Autodesk Fusion 360 part; units mm, degrees
sketch "Sketch1" plane through (0, 0, 0) normal (0, 0, 1) x (1, 0, 0)
  line L0 (0, 0) -> (50.8, 0)
  line L1 (50.8, 0) -> (50.8, 50.8)
  line L2 (50.8, 50.8) -> (0, 50.8)
  line L3 (0, 50.8) -> (0, 0)
  dimension "d1" = 50.8
  dimension "d2" = 50.8
extrude "Extrude1" add sketch "Sketch1" along normal blind 31.75
sketch "Sketch2" plane through (50.8, 0, 0) normal (1, 0, 0) x (0, 1, 0)
  line L0 (0, 0) -> (50.8, 0)
  line L1 (50.8, 0) -> (50.8, 31.75)
  line L2 (50.8, 31.75) -> (0, 31.75)
  line L3 (0, 31.75) -> (0, 0)
  line L4 (50.8, 23.368) -> (10.16, 23.368)
  line L5 (10.16, 23.368) -> (10.16, 3.81)
  line L6 (10.16, 3.81) -> (50.8, 3.81)
  line L7 (50.8, 3.81) -> (50.8, 23.368)
  dimension "d5" = 40.64
  dimension "d6" = 19.558
  dimension "d14" = 3.81
extrude "Extrude2" cut sketch "Sketch2" against normal blind 40.64 contours L1 L4 L5 L6 L7
sketch "Sketch3" plane through (0, 0, 31.75) normal (0, 0, 1) x (-1, 0, 0)
  line L0 (0, -50.8) -> (0, 0)
  line L1 (0, 0) -> (-50.8, 0)
  line L2 (-50.8, 0) -> (-50.8, -50.8)
  line L3 (-50.8, -50.8) -> (0, -50.8)
  line L4 (0, 0) -> (-25.4, 0)
  line L5 (-25.4, 0) -> (-25.4, -25.4)
  line L6 (-25.4, -25.4) -> (0, -25.4)
  line L7 (0, -25.4) -> (0, 0)
  dimension "d10" = 25.4
  dimension "d11" = 25.4
extrude "Extrude3" add sketch "Sketch3" along normal blind 152.4 contours L0 L1 L4 L5 L6 L7
fillet "Fillet1" radius 2.54 2 edges at (25.4, 12.7, 31.75) (12.7, 25.4, 31.75)
sketch "Sketch4" plane through (0, 0, 0) normal (0, 0, -1) x (1, 0, 0)
  line L0 (0, 0) -> (0, -50.8)
  line L1 (0, -50.8) -> (50.8, -50.8)
  line L2 (50.8, -50.8) -> (50.8, 0)
  line L3 (50.8, 0) -> (0, 0)
  line L4 (2.54, -2.54) -> (22.86, -2.54)
  line L5 (22.86, -2.54) -> (22.86, -22.86)
  line L6 (22.86, -22.86) -> (2.54, -22.86)
  line L7 (2.54, -22.86) -> (2.54, -2.54)
  dimension "d17" = 2.54
  dimension "d18" = 2.54
  dimension "d19" = 20.32
  dimension "d20" = 20.32
sketch "Sketch5" plane through (0, 0, 0) normal (0, 0, -1) x (1, 0, 0)
  line L0 (5.08, -5.08) -> (20.32, -5.08)
  line L1 (20.32, -5.08) -> (20.32, -20.32)
  line L2 (20.32, -20.32) -> (5.08, -20.32)
  line L3 (5.08, -20.32) -> (5.08, -5.08)
  line L4 (2.54, -2.54) -> (22.86, -2.54)
  line L5 (2.54, -22.86) -> (2.54, -2.54)
  dimension "d21" = 2.54
  dimension "d22" = 2.54
  dimension "d23" = 15.24
  dimension "d24" = 15.24
extrude "Extrude4" add sketch "Sketch5" along normal blind 5.08
loft "Loft1" add profiles "Sketch4" section 1 contours L4 L5 L6 L7 section 2 face at (10.16, 15.24, -5.08)
sketch "Sketch6" plane through (0, 0, 184.15) normal (0, 0, 1) x (-1, 0, 0)
  line L0 (0, -25.4) -> (0, 0)
  line L1 (0, 0) -> (-25.4, 0)
  line L2 (-25.4, 0) -> (-25.4, -25.4)
  line L3 (-25.4, -25.4) -> (0, -25.4)
  line L4 (-2.54, -22.86) -> (-22.86, -22.86)
  line L5 (-22.86, -22.86) -> (-22.86, -2.54)
  line L6 (-22.86, -2.54) -> (-2.54, -2.54)
  line L7 (-2.54, -2.54) -> (-2.54, -22.86)
  line L8 (-5.08, -20.32) -> (-20.32, -20.32)
  line L9 (-20.32, -20.32) -> (-20.32, -5.08)
  line L10 (-20.32, -5.08) -> (-5.08, -5.08)
  line L11 (-5.08, -5.08) -> (-5.08, -20.32)
  dimension "d27" = 2.54
  dimension "d28" = 2.54
  dimension "d29" = 2.54
  dimension "d30" = 20.32
  dimension "d31" = 2.54
  dimension "d32" = 15.24
  dimension "d33" = 15.24
  dimension "d34" = 2.54
extrude "Extrude5" cut sketch "Sketch6" against normal blind 5.08 contours L8 L9 L10 L11
loft "Loft2" cut profiles "Sketch6" section 1 contours L4 L5 L6 L7 section 2 face at (15.24, 15.24, 179.07)
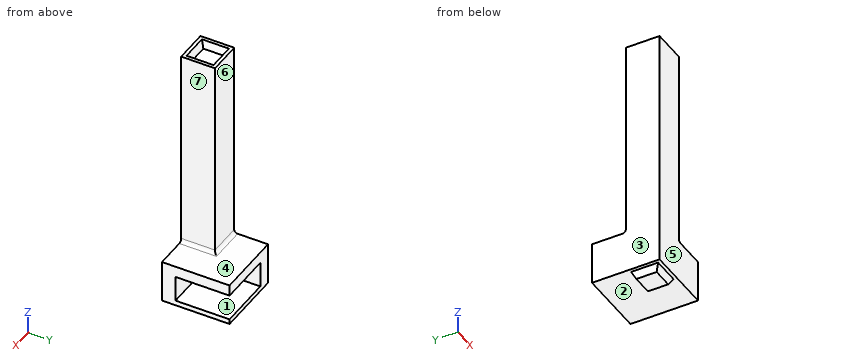
The listing builds one solid part. Answer for the finished solid, in the listing's coordinates (mm). Face numbers are marked on the shaded views. A direction names the side the tool comes from. Coordinates: 2 decimals unless noted, no trailing zeros. Loops run counter-clockwise (first coordinate to the right, second up) from the corner with the lowest first, then second, coordinate; pieces in that order, holes last. Notation, with made-up numbers: M 53.25,49.25 L 86.25,49.25 A10 ccw 86.25,60.25 Z; hole C 37,-26.5 d1. An arc over 180 degrees is marked long. Answer as a JSON object with one key per item and string values. Group by question number.
Item 1: Determine the mould class of the marked faces 1, 2, 3 and 4 for opening direction Z: +Z half, -Z half, draft (parallel to the pull), parting line (faces both ways), or undercut.
Item 2: Each of these flat-tipped pins is pushed along its axis until it touches: P1, Ø20.5, axis at y = 8.5, z = 134.5, coming from the +X side; P2, Ø10, axis at x = 43.5, y = 6, coming from the -Z side; P3, Ø12, axis at x = 16, y = 13, coming from the +Z side. Where does it stop, or does it pass through?
Item 3: Section C-C (z = 156) is taken. Write down the section's boundary in (x, y).
Item 4: Which of the six approach directions +Z, -Z, +X, -X, +Y, -Y give full straight-line access (tool end or side, diameter ignored) to the marked faces 5, 6 and 7?
Item 5: Consider L1, parallel to Z at x = 13, y = 19; L2, parallel to Z at x = 32.5, y = 29.5; L3, parallel to X at y = 7, z = 133. Determine where each line is inside the solid, lowest interval first.
Item 6: Section A-A (x = 37) is taken. Write down the section's boundary in (y, z), and give its area (3 significant figures).
Solved:
{
 "1": {"face 1": "undercut", "face 2": "-Z half", "face 3": "draft", "face 4": "+Z half"},
 "2": {"P1": "stops at x = 25.4", "P2": "stops at z = 0", "P3": "stops at z = 182.43"},
 "3": {"outline": "M 0,0 L 25.4,0 L 25.4,25.4 L 0,25.4 Z"},
 "4": {"face 5": "+Z, -Z, +X, -X, -Y", "face 6": "+Z, +X, -X, +Y", "face 7": "+Z, +X, +Y, -Y"},
 "5": {"L1": "z = -5.08 to 3.81, 23.37 to 179.07", "L2": "z = 0 to 3.81, 23.37 to 31.75", "L3": "x = 0 to 25.4"},
 "6": {"outline": "M 0,0 L 50.8,0 L 50.8,3.81 L 10.16,3.81 L 10.16,23.37 L 50.8,23.37 L 50.8,31.75 L 0,31.75 Z", "area": "818 mm2"}
}
